The listing builds one solid part. Answer for the finished solid, in the listing's coordinates (mm). A direction names the side the tool comes from. Round coordinates to 2 decimals unless told otherwise and drop trailing zeros. Loops run counter-clockwise (first coordinate to the right, second up) from the corner with the lowest first, then second, coordinate; pieces in that order, holes last. Notation, with made-up numbers: (58, 66.5) -> (63, 66.5) arc R18 ccw to (63, 80.5) -> close; hole circle Ø7 at (58, 10.5). An arc over 180 degrees is marked (long way). Use a Markdown table: item, result. Add a question column.
Q1. Section A-A on z = 8 is taken. Give the vertices of the cut face in (x, y), then the cut area to 3 significant figures.
Q2. Given pin 1 Ø1 at (x, y) = (4.5, 1) entering from +Z; pin 2 Ø1.1 at (x, z) = (0, -12.6) entering from +Y; pin 3 Ø2 at (x, y) = (2.5, 2) entering from +Z, each flat-ended and moving along its own axis, determine where each tip first touches the part or whether it passes through.
Q3. Section C-C on z = 0 is taken. Give the vertices of the cut face in (x, y).
Q4. Which of the six approach directions +Z, -Z, +X, -X, +Y, -Y give full straight-line access (tool end or side, diameter ignored) to faces 1 (the cylindrical face through (-0.13, 3.496, -13.186)), 2 (the flat face through (-7, 3.2, 10)), 3 (the cylindrical face through (-0.238, 1.927, 9.074))?
Q5. Section B-B on x = -8.75 is taken. Give the vertices of the cut face in (y, z), then the cut area to 3 significant figures.
Q6. For a pull along Y with two mould halves and no side action, classify faces 4 (the cylindrical face through (-5.8, 1.927, -6.748)), 5 (the flat face through (-10, 0.6, 7)), 6 (the flat face through (-6, 3.8, 0)) as released by +Y, released by -Y, zero draft, split by the parting line, or undercut.
Q7. Consider line 1 (X direction, y = 1.9, z = 0); line 2 (Y direction, x = -9.5, z = 9.75). Determine where each line is inside the solid, lowest interval first.
Q8. Section D-D on y = 2.2 is taken. Give the number of separate pieces and of enclosed holes in the cut face, then the cut area to 3 significant figures.
Autodesk Inventor part; units mm, degrees
ref_plane "YZ Plane" through (0, 0, 0) normal (1, 0, 0) x (0, 1, 0)
ref_plane "XZ Plane" through (0, 0, 0) normal (0, 1, 0) x (-1, 0, 0)
ref_plane "XY Plane" through (0, 0, 0) normal (0, 0, 1) x (1, 0, 0)
sketch "Sketch1" plane through (0, 0, 0) normal (0, 1, 0) x (-1, 0, 0)
  circle A0 centre (0, 0) radius 15
  dimension "d0" = 30
extrude "Extrusion1" add sketch "Sketch1" along normal blind 3.8
sketch "Sketch2" plane through (0, 3.8, 0) normal (0, 1, 0) x (1, 0, 0)
  circle A0 centre (0, 0) radius 8 construction
  circle A1 centre (-8, 0) radius 1.1
  circle A2 centre (-5.6569, -5.6569) radius 1.1
  circle A3 centre (0, -8) radius 1.1
  circle A4 centre (5.6569, -5.6569) radius 1.1
  circle A5 centre (8, 0) radius 1.1
  circle A6 centre (5.6569, 5.6569) radius 1.1
  circle A7 centre (0, 8) radius 1.1
  circle A8 centre (-5.6569, 5.6569) radius 1.1
  circle A9 centre (0, 0) radius 5.5
  dimension "d3" = 16
  dimension "d4" = 2.2
  dimension "d7" = 360
  dimension "d9" = 11
extrude "Extrusion2" cut sketch "Sketch2" against normal through all
sketch "Sketch3" plane through (0, 0, 0) normal (1, 0, 0) x (0, 1, 0)
  point P0 (0, 0)
sketch "Sketch4" plane through (0, 0, 0) normal (1, 0, 0) x (0, 1, 0)
  line L0 (3.8, 5.5) -> (0, 5.5) construction
  line L1 (0, 5.5) -> (0, 6.9) construction
  line L2 (0, 6.9) -> (3.8, 6.9) construction
  line L3 (3.8, 6.9) -> (3.8, 5.5) construction
  line L4 (0, -5.5) -> (3.8, -5.5) construction
  line L5 (3.8, -5.5) -> (3.8, -6.9) construction
  line L6 (3.8, -6.9) -> (0, -6.9) construction
  line L7 (0, -6.9) -> (0, -5.5) construction
  line L8 (0, 15) -> (3.8, 15) construction
  line L9 (3.8, 15) -> (3.8, 9.1) construction
  line L10 (3.8, 9.1) -> (0, 9.1) construction
  line L11 (0, 9.1) -> (0, 15) construction
  line L12 (3.8, -15) -> (0, -15) construction
  line L13 (0, -15) -> (0, -9.1) construction
  line L14 (0, -9.1) -> (3.8, -9.1) construction
  line L15 (3.8, -9.1) -> (3.8, -15) construction
  line L16 (0.6, -15) -> (3.2, -15)
  line L17 (3.2, -15) -> (3.2, -12)
  line L18 (3.2, -12) -> (0.6, -12)
  line L19 (0.6, -12) -> (0.6, -15)
  line L20 (-0.76, 0) -> (4.56, 0)
  point P0 (0, 0)
  point P1 (1.9, -15)
  dimension "d12" = 0.6
  dimension "d15" = 12
revolve "Revolution1" cut sketch "Sketch4" angle 360 about axis through (0, -10, 0) along (0, 1, 0)
sketch "Sketch5" plane through (0, 3.2, 0) normal (0, -1, 0) x (1, 0, 0)
  circle A0 centre (0, -12.6) radius 0.6
  circle A1 centre (0, 0) radius 12 construction
  circle A2 centre (0, 0) radius 15 construction
  circle A3 centre (-8, 0) radius 1.1 construction
  circle A4 centre (8, 0) radius 1.1 construction
  circle A5 centre (5.6569, 5.6569) radius 1.1 construction
  circle A6 centre (-5.6569, -5.6569) radius 1.1 construction
  circle A7 centre (-5.6569, 5.6569) radius 1.1 construction
  circle A8 centre (5.6569, -5.6569) radius 1.1 construction
  circle A9 centre (0, 8) radius 1.1 construction
  circle A10 centre (0, -8) radius 1.1 construction
  circle A11 centre (0, 0) radius 5.5 construction
  dimension "d17" = 1.2
extrude "Extrusion3" cut sketch "Sketch5" against normal up to surface (0.6 mm away)
properties part number "Pully_r12"
Checked values:
| question | item | result |
|---|---|---|
| 1 | outline | (-12.69, 0) -> (-1.1, 0) -> (-1.1, 3.8) -> (-12.69, 3.8) -> (-12.69, 3.2) -> (-8.94, 3.2) -> (-8.94, 0.6) -> (-12.69, 0.6) -> close; (1.1, 0) -> (12.69, 0) -> (12.69, 0.6) -> (8.94, 0.6) -> (8.94, 3.2) -> (12.69, 3.2) -> (12.69, 3.8) -> (1.1, 3.8) -> close |
| 1 | area | 68.6 mm2 |
| 2 | pin 1 | stops at z = 14.4 |
| 2 | pin 2 | stops at y = 0.6 |
| 2 | pin 3 | stops at z = 11.91 |
| 3 | outline | (-15, 0) -> (-9.1, 0) -> (-9.1, 3.8) -> (-15, 3.8) -> (-15, 3.2) -> (-12, 3.2) -> (-12, 0.6) -> (-15, 0.6) -> close; (-6.9, 0) -> (-5.5, 0) -> (-5.5, 3.8) -> (-6.9, 3.8) -> close; (5.5, 0) -> (6.9, 0) -> (6.9, 3.8) -> (5.5, 3.8) -> close; (9.1, 0) -> (15, 0) -> (15, 0.6) -> (12, 0.6) -> (12, 3.2) -> (15, 3.2) -> (15, 3.8) -> (9.1, 3.8) -> close |
| 4 | face 1 | +Y |
| 4 | face 2 | none |
| 4 | face 3 | +Y, -Y |
| 5 | outline | (0, -12.18) -> (0.6, -12.18) -> (0.6, -8.21) -> (3.2, -8.21) -> (3.2, -12.18) -> (3.8, -12.18) -> (3.8, -0.8) -> (0, -0.8) -> close; (0, 0.8) -> (3.8, 0.8) -> (3.8, 12.18) -> (3.2, 12.18) -> (3.2, 8.21) -> (0.6, 8.21) -> (0.6, 12.18) -> (0, 12.18) -> close |
| 5 | area | 65.8 mm2 |
| 6 | face 4 | zero draft |
| 6 | face 5 | undercut |
| 6 | face 6 | released by +Y |
| 7 | line 1 | x = -12 to -9.1, -6.9 to -5.5, 5.5 to 6.9, 9.1 to 12 |
| 7 | line 2 | y = 0 to 0.6, 3.2 to 3.8 |
| 8 | separate pieces | 1 |
| 8 | enclosed holes | 9 |
| 8 | area | 327 mm2 |
